from build123d import *

# Parameters (mm, degrees)
F0_W         = 25
F0_H         = 35
F1_DEPTH     = 15
F2_R         = 1.75
F3_DEPTH     = 25
F4_W         = 9.5
F4_H         = 20
F5_DEPTH     = 15
F6_R         = 1.75
F7_DEPTH     = 4
F8_R         = 2.3
F9_DEPTH     = 15
F10_R        = 3
F10_R_2      = 2.3
F11_DEPTH    = 5
F12_T1_DEPTH = 55.8601958556


# Not quite as in the source:
# - a fillet or chamfer that OpenCascade refuses, or shapes differently, is made with other operations: its cross-section is extruded or revolved along the edge and cut away or added


with BuildPart() as f1:
    # F0 (on Top) → F1 (new body)
    with BuildSketch(Plane.XY):
        Rectangle(F0_W, F0_H)
    extrude(amount=-F1_DEPTH)

    # F2 (on face) → F3 (cut)
    with BuildSketch(Plane.YZ.offset(12.5)):
        with Locations((0, -4)):
            Circle(F2_R)
    extrude(amount=-F3_DEPTH, mode=Mode.SUBTRACT)

    # F4 (on face) → F5 (cut)
    with BuildSketch(Plane.XY):
        Rectangle(F4_W, F4_H)
    extrude(amount=-F5_DEPTH, mode=Mode.SUBTRACT)

    # F6 (on face) → F7 (cut)
    with BuildSketch(Plane(origin=(-12.5, 0, 0), x_dir=(0, -1, 0), z_dir=(-1, 0, 0))):
        Polygon((-2.8, -2.3834192463), (-2.8, -5.6165807537), (0, -7.2331615075), (2.8, -5.6165807537), (2.8, -2.3834192463), (0, -0.7668384925), align=None)
        with Locations((0, -4)):
            Circle(F6_R, mode=Mode.SUBTRACT)
    extrude(amount=-F7_DEPTH, mode=Mode.SUBTRACT)

    # F8 (on face) → F9 (cut)
    with BuildSketch(Plane.XY):
        with Locations((-8, 13.5)):
            Circle(F8_R)
        with Locations((8, 13.5)):
            Circle(F8_R)
        with Locations((8, -13.5)):
            Circle(F8_R)
        with Locations((-8, -13.5)):
            Circle(F8_R)
    extrude(amount=-F9_DEPTH, mode=Mode.SUBTRACT)

    # F10 (on face) → F11 (cut)
    with BuildSketch(Plane(origin=(0, 0, -15), x_dir=(1, 0, 0), z_dir=(0, 0, -1))):
        with Locations((-8, 13.5)):
            Circle(F10_R)
        with Locations((-8, 13.5)):
            Circle(F10_R_2, mode=Mode.SUBTRACT)
        with Locations((8, 13.5)):
            Circle(F10_R)
        with Locations((8, 13.5)):
            Circle(F10_R_2, mode=Mode.SUBTRACT)
        with Locations((8, -13.5)):
            Circle(F10_R)
        with Locations((8, -13.5)):
            Circle(F10_R_2, mode=Mode.SUBTRACT)
        with Locations((-8, -13.5)):
            Circle(F10_R)
        with Locations((-8, -13.5)):
            Circle(F10_R_2, mode=Mode.SUBTRACT)
    extrude(amount=-F11_DEPTH, mode=Mode.SUBTRACT)

    # F12: chamfer of 6 on 1 edges, made by hand

    # F12_s2 → F12_t1 (cut)
    with BuildSketch(Plane.YZ.offset(-27.9300979278)):
        Polygon((17.5, -6), (11.5, 0), (17.5, 0), align=None)
    extrude(amount=F12_T1_DEPTH, mode=Mode.SUBTRACT)


solid = f1.part
Input: part model. Units: mm. Frame: model coordinates. A direction names the side the tool comes from. Give positions to 0.01 mm unless a question says otherwise; leave off trailing zeros. Write each loop counter-clockwise with the first axis right and the second up, starting at its lowest first coordinate (ties: lowest second). Pieces come first, ordered by that corner, then holes. Notation, with made-up numbers: M 39.5,65 L 92.5,65 A11 ccw 92.5,77 Z; hole C 22.25,28.5 d10. An arc over 180 degrees is marked long. Use one line per item in the form item = value.
1. Reachability of faces 4 (the face through (5, 0, -15)), 5 (the face through (0, 10, -7)), 6 (the face through (-6.616, 16.162, -12.535)), 7 (the face through (-8.5, 1.3, -5.4)) from +Z, -Z, +X, -X, +Y, -Y: full face, straight path, thin tool, end or side. Return the list, or none.
Outcome:
face_4 = -Z, +X, -X, +Y, -Y
face_5 = +Z, -Z
face_6 = -Z
face_7 = -X
2. Ray query, L1, parallel to X at y = 13.5, z = -11.3; L2, parallel to Y at x = 8, z = -6; L3, parallel to X at y = -13.5, z = -3. Return the intervals inside material, ascending.
Outcome:
L1 = -12.5 to -11, -5 to 5, 11 to 12.5
L2 = -17.5 to -15.8, -11.2 to 11.2, 15.8 to 17.5
L3 = -12.5 to -10.3, -5.7 to 5.7, 10.3 to 12.5
3. First-contact query: P1, Ø5.5, axis at x = -8, y = 13.5, coming from the +Z side; P2, Ø3, axis at x = 7.5, y = -12.5, coming from the -Z side; P3, Ø3.5, axis at x = -11.5, z = -3.5, coming from the +Y side. Flat tips, straight axial feed; report the tip coordinate or a pass-through.
Outcome:
P1 = 0
P2 = -10
P3 = 16.75
4. Cut plane C-C on z = -9.5. Return loops of the section in (x, y), and give its area (3 significant figures).
Outcome:
outline = M -12.5,-17.5 L 12.5,-17.5 L 12.5,17.5 L -12.5,17.5 Z; hole C -8,-13.5 d4.6; hole C -8,13.5 d4.6; hole M -4.75,-10 L 4.75,-10 L 4.75,10 L -4.75,10 Z; hole C 8,-13.5 d4.6; hole C 8,13.5 d4.6
area = 619 mm²
5. Cut plane A-A on x = -8. Return loops of the section in (y, z).
Outcome:
outline = M -17.5,-15 L -16.5,-15 L -16.5,-10 L -15.8,-10 L -15.8,0 L -17.5,0 Z; M -11.2,-10 L -10.5,-10 L -10.5,-15 L 10.5,-15 L 10.5,-10 L 11.2,-10 L 11.2,0 L -11.2,0 Z; M 15.8,-10 L 16.5,-10 L 16.5,-15 L 17.5,-15 L 17.5,-6 L 15.8,-4.3 Z; hole C 0,-4 d3.5
6. Mould query, pull axis Z, two halves, no side actions, for faces 1 (the face through (-11, -2.8, -4)), 2 (the face through (7, -11, -10)), 3 (the face through (-6, -3, 0)). Classes: released by +Z, released by -Z, zero draft, split by the parting line, or undercut.
Outcome:
face_1 = undercut
face_2 = released by -Z
face_3 = released by +Z
7. Cut plane D-D on x = 4. Return loops of the section in (y, z), and give its area (3 significant figures).
Outcome:
outline = M -17.5,-15 L -10,-15 L -10,0 L -17.5,0 Z; M 10,-15 L 17.5,-15 L 17.5,-6 L 11.5,0 L 10,0 Z
area = 207 mm²
8. Cut plane B-B on y = -13.5. Return loops of the section in (x, z).
Outcome:
outline = M -12.5,-15 L -11,-15 L -11,-10 L -10.3,-10 L -10.3,0 L -12.5,0 Z; M -5.7,-10 L -5,-10 L -5,-15 L 5,-15 L 5,-10 L 5.7,-10 L 5.7,0 L -5.7,0 Z; M 10.3,-10 L 11,-10 L 11,-15 L 12.5,-15 L 12.5,0 L 10.3,0 Z
